```python
from build123d import *

# Parameters (mm, degrees)
CUT_EXTRUDE_1_DEPTH      = 86.422479477
CUT_EXTRUDE_1_DEPTH_BACK = 86.422479477
SKETCH_3_R               = 1.5
CHAMFER_1_SIZE           = 2


# Read off the part's stored shape, not the designer's step: M12 机械螺纹 螺柱1
with BuildPart() as part:
    # 草图1 → 旋转1 (revolve)
    with BuildSketch(Plane.XY, mode=Mode.PRIVATE) as revolve_1_sk:
        Polygon((0, 0), (2.309401077, 4), (9.5, 4), (9.5, 6), (26.2, 6), (26.2, 5), (28.2, 5), (28.2, 6), (72.2, 6), (72.2, 4), (85, 4), (85, 0), align=None)
    revolve(revolve_1_sk.sketch.rotate(Axis((85, 0, 0), (-1, 0, 0)), 90), axis=Axis((85, 0, 0), (-1, 0, 0)))

    # M12 机械螺纹 螺柱1 outline → M12 机械螺纹 螺柱1 (revolve, cut)
    with BuildSketch(Plane.YX):
        Polygon((6, 72.2), (5.053, 72.2), (6, 71.253), align=None)
    revolve(axis=Axis((0, 0, 0), (1, 0, 0)), mode=Mode.SUBTRACT)

    # 草图3 → 切除-拉伸1 (cut, two sides: drawn at the far end of the back side and taken through both)
    with BuildSketch(Plane.XY.offset(-CUT_EXTRUDE_1_DEPTH_BACK)):
        with Locations((80.2, 0)):
            Circle(SKETCH_3_R)
    extrude(amount=CUT_EXTRUDE_1_DEPTH + CUT_EXTRUDE_1_DEPTH_BACK, mode=Mode.SUBTRACT)

    # 倒角1
    chamfer_1_edges = [part.edges().sort_by_distance(p)[0] for p in [
        (9.5, 0, 6),
    ]]
    chamfer(chamfer_1_edges, length=CHAMFER_1_SIZE - 0.0001)  # a hair under: the kernel refuses the full size


solid = part.part
```
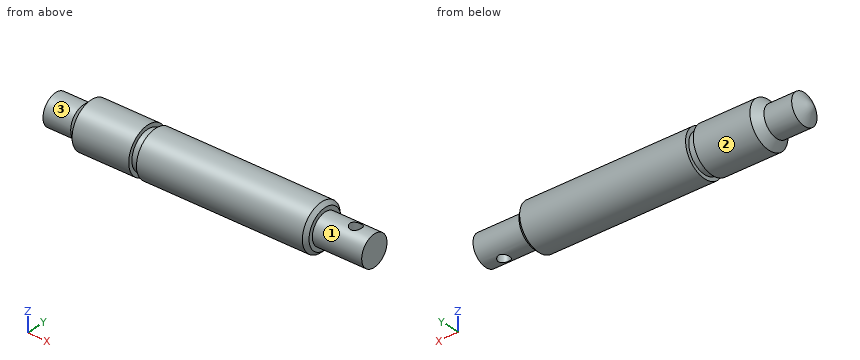
Geometry: final body of the model. Coordinates: model frame, mm. Face numbers are marked on the shaded views. A direction names the side the tool comes from. Round coordinates to 2 decimals unless told otherwise and drop trailing zeros. Write each loop counter-clockwise with the first axis right and the second up, starting at its lowest first coordinate (ties: lowest second). Pieces come first, ordered by that corner, then holes. Notation, with made-up numbers: (29, 5) -> (80, 5) arc R17 cw to (80, 10) -> close; hole circle Ø4 at (18.25, 76.25). An arc over 180 degrees is marked (long way). Use CSV: the item, a comma, the result in double quotes. Start each with the question number.
Q1. First-contact query: pin 1 Ø3.5 at (x, y) = (80.2, 0) entering from +Z; pin 2 Ø1.5 at (y, z) = (-1, -1) entering from -X; pin 3 Ø1.5 at (x, z) = (32, 4.5) entering from -Y. Flat tips, straight axial feed; report the tip coordinate or a pass-through.
Q2. Line query: L1, parallel to Z at x = 75, y = -0.25; L2, parallel to Y at x = 67, z = 3.25; L3, parallel to X at y = -5.5, z = 2. Output: solid intervals per line, ascending.
Q3. Section B-B (x = 40.5). Return loops of the section in (y, z).
Q4. Reachability of the marked faces 1, 2 and 3 from +Z, -Z, +X, -X, +Y, -Y: full face, straight path, thin tool, end or side. Return the list, or none.
Q5. Section A-A (x = 79.5). Return loops of the section in (y, z), plus the area to 3 significant figures.
Result sheet:
1,pin 1,"z = 4"
1,pin 2,"x = 0.38"
1,pin 3,"y = -4.68"
2,L1,"-3.99 to 3.99"
2,L2,"-5.04 to 5.04"
2,L3,"11.35 to 26.2, 28.2 to 71.4"
3,outline,"circle Ø12 at (0, 0)"
4,face 1,"+X"
4,face 2,"+X, -X"
4,face 3,"-X"
5,outline,"(-1.33, -3.77) -> (-1.33, 3.77) arc R4 ccw to start; (1.33, -3.77) arc R4 ccw to (1.33, 3.77) -> close"
5,area,"29.4 mm²"
